Verification items for this drawing (mm, ordinates from the low corner). A direction names the side the tool comes from. Round coordinates to 2 decimals unless told otherwise and drop trailing zeros. Loops run counter-clockwise (first coordinate to the right, second up) from the corner with the lowest first, then second, coordinate; pieces in that order, holes last. Notation, with made-up numbers: (-10.75, -22.75) - (0.25, -22.75) arc R14 cw to (0.25, -12.75) - close; hole circle Ø11 at (-1, -36.75). An arc over 180 degrees is marked (long way). Put each result on its own line as item: value.
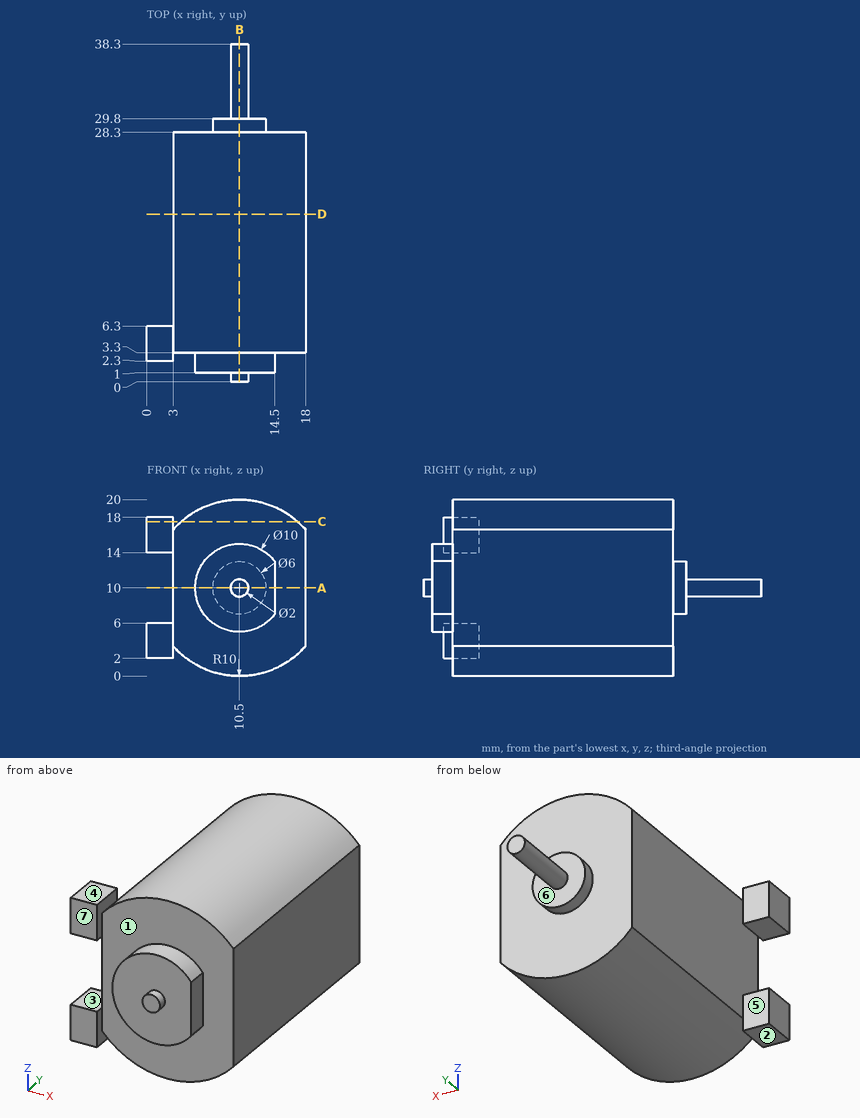
Item 1: Section check B-B on x = 10.5. Enter the section's corners in (y, z).
Filled sheet:
outline: (0, 9) - (1, 9) - (1, 5) - (3.3, 5) - (3.3, 0) - (28.3, 0) - (28.3, 7) - (29.8, 7) - (29.8, 9) - (38.3, 9) - (38.3, 11) - (29.8, 11) - (29.8, 13) - (28.3, 13) - (28.3, 20) - (3.3, 20) - (3.3, 15) - (1, 15) - (1, 11) - (0, 11) - close
Item 2: Section check D-D on y = 19. Enter the section's corners in (x, z).
Filled sheet:
outline: (3, 3.39) arc R10 ccw to (18, 3.39) - (18, 16.61) arc R10 ccw to (3, 16.61) - close
Item 3: Go/stop test with flat-tipped pins: pin 1 (3.5 mm diameter, centred on x = 1.5, z = 4, fed in from +Y); pin 2 (0.9 mm diameter, centred on x = 2, z = 16, fed in from +Y); pin 3 (6 mm diameter, centred on x = 3, y = 6, fed in from +Z). Record where each tip stops, or that it passes through.
Filled sheet:
pin 1: y = 28.3
pin 2: y = 6.3
pin 3: z = 18.93
Item 4: Release check for a two-part mould opening along Z. For the marked faces 1, 2 and 3 record: +Z half, -Z half, draft (parallel to the pull), parting line (faces both ways), or undercut.
Filled sheet:
face 1: draft
face 2: -Z half
face 3: undercut
Item 5: Section check A-A on z = 10. Enter the section's corners in (x, y), then the cut area to 3 significant figures.
Filled sheet:
outline: (3, 3.3) - (5.5, 3.3) - (5.5, 1) - (9.5, 1) - (9.5, 0) - (11.5, 0) - (11.5, 1) - (14.5, 1) - (14.5, 3.3) - (18, 3.3) - (18, 28.3) - (13.5, 28.3) - (13.5, 29.8) - (11.5, 29.8) - (11.5, 38.3) - (9.5, 38.3) - (9.5, 29.8) - (7.5, 29.8) - (7.5, 28.3) - (3, 28.3) - close
area: 424 mm²
Item 6: Thickness scan on line 1 (X direction, y = 6, z = 12.5); line 2 (Y direction, x = 7.75, z = 8.25); line 3 (Y direction, x = 1.5, z = 2.25). Record the ranges inside material, lowest first. Write a range as from..to.
Filled sheet:
line 1: 3..18
line 2: 1..28.3
line 3: 2.3..6.3
Item 7: Tool access check on the marked faces 4, 5, 6 and 7. Record the directions out of +Z, -Z, +X, -X, +Y, -Y that give a thin tool (end or side, any length) a straight path to the whole face; none if there is none.
Filled sheet:
face 4: +Z, -X, +Y, -Y
face 5: +Z, -Z, -X, +Y
face 6: +Y
face 7: +Z, -Z, -X, -Y
Item 8: Section check C-C on z = 17.5. Enter the section's corners in (x, y).
Filled sheet:
outline: (0, 2.3) - (3, 2.3) - (3, 6.3) - (0, 6.3) - close; (3.89, 3.3) - (17.11, 3.3) - (17.11, 28.3) - (3.89, 28.3) - close
